The listing builds one solid part. Answer for the finished solid, in the listing's coordinates (mm). A direction names the side the tool comes from. Give positions to 0.01 mm unless a question says otherwise; leave off trailing zeros. Write each loop counter-clockwise with the first axis right and the second up, starting at its lowest first coordinate (ties: lowest second). Pieces come first, ordered by that corner, then holes. Notation, with made-up numbers: (-6, 75.5) - (15, 75.5) arc R24 cw to (15, 112.5) - close; hole circle Ø9 at (61, 80.5). An arc over 180 degrees is marked (long way). Return JSON: item names as keys, results as strings.
from build123d import *

# Parameters (mm, degrees)
SKETCH_1_W           = 20
SKETCH_1_H           = 19
SKETCH_1_R           = 7.5
EXTRUDE_3_DEPTH      = 5
EXTRUDE_4_DEPTH      = 0.0001
EXTRUDE_4_DEPTH_BACK = 5
SKETCH_3_W           = 5
SKETCH_3_H           = 2
SKETCH_4_R           = 1.5
CUT_EXTRUDE_1_DEPTH  = 25.718414189
SKETCH_5_R           = 1.5
CUT_EXTRUDE_2_DEPTH  = 25.718414189
SKETCH_6_W           = 5.334039958
SKETCH_6_H           = 1
CUT_EXTRUDE_3_DEPTH  = 19.445893852


with BuildPart() as part:
    # 草图1 → 凸台-拉伸3 (new body)
    with BuildSketch(Plane(origin=(0, 0, 0), x_dir=(0, 0, -1), z_dir=(1, 0, 0))):
        Rectangle(SKETCH_1_W, SKETCH_1_H)
        Circle(SKETCH_1_R, mode=Mode.SUBTRACT)
    extrude(amount=EXTRUDE_3_DEPTH)

    # 草图3 → 凸台-拉伸4 (add, two sides: drawn at the far end of the back side and taken through both)
    with BuildSketch(Plane.ZY.offset(-EXTRUDE_4_DEPTH_BACK)):
        with Locations((12.5, 8.5)):
            Rectangle(SKETCH_3_W, SKETCH_3_H)
        with Locations((12.5, -8.5)):
            Rectangle(SKETCH_3_W, SKETCH_3_H)
        with Locations((-12.5, 8.5)):
            Rectangle(SKETCH_3_W, SKETCH_3_H)
        with Locations((-12.5, -8.5)):
            Rectangle(SKETCH_3_W, SKETCH_3_H)
    extrude(amount=EXTRUDE_4_DEPTH + EXTRUDE_4_DEPTH_BACK)

    # 草图4 → 切除-拉伸1 (cut, through all)
    with BuildSketch(Plane(origin=(0, 9.5, 0), x_dir=(1, 0, 0), z_dir=(0, 1, 0))):
        with Locations(Location((2.49995, -12.5, 0), (0, 0, 270))):
            Circle(SKETCH_4_R)
    extrude(amount=-CUT_EXTRUDE_1_DEPTH, mode=Mode.SUBTRACT)

    # 草图5 → 切除-拉伸2 (cut, through all)
    with BuildSketch(Plane(origin=(0, 9.5, 0), x_dir=(1, 0, 0), z_dir=(0, 1, 0))):
        with Locations(Location((2.49995, 12.5, 0), (0, 0, 270))):
            Circle(SKETCH_5_R)
    extrude(amount=-CUT_EXTRUDE_2_DEPTH, mode=Mode.SUBTRACT)

    # 草图6 → 切除-拉伸3 (cut, through all)
    with BuildSketch(Plane(origin=(5, 0, 0), x_dir=(0, 0, -1), z_dir=(1, 0, 0))):
        with Locations((-7.5, 0)):
            Rectangle(SKETCH_6_W, SKETCH_6_H)
    extrude(amount=-CUT_EXTRUDE_3_DEPTH, mode=Mode.SUBTRACT)


solid = part.part
Item 1: A cutting plane is placed at B-B on x = 3. Give the number of separate pieces and of enclosed holes in the cut face, then the cut area to 3 significant figures.
Answer below:
{"separate pieces": "5", "enclosed holes": "0", "area": "218 mm²"}
Item 2: A cutting plane is placed at A-A on z = 4.5. Determine the outline of the cut face in (x, y).
Answer below:
{"outline": "(0, -9.5) - (5, -9.5) - (5, -6) - (0, -6) - close; (0, 6) - (5, 6) - (5, 9.5) - (0, 9.5) - close"}
Item 3: Consider L1, parallel to X at y = -8.6, z = 12.5; L2, parallel to Y at x = 3.75, z = 8; L3, parallel to Z at x = 3.4, y = 8.75. Determine where each line is inside the solid, lowest interval first.
Answer below:
{"L1": "x = 0 to 1, 4 to 5", "L2": "y = -9.5 to -0.5, 0.5 to 9.5", "L3": "z = -15 to -13.7, -11.3 to 11.3, 13.7 to 15"}
Item 4: The mould has two halves that part along X. Classify faces 4 (the face through (0, -8, -13)), 5 (the face through (2.57, -8.49, 11)), 6 (the face through (3, 0.5, 9)): +X half, -X half, draft (parallel to the pull), parting line (faces both ways), or undercut.
Answer below:
{"face 4": "-X half", "face 5": "undercut", "face 6": "draft"}
Item 5: For faces 1 (the face through (2, 0, -10)), 2 (the face through (0, -8, 12)), 3 (the face through (4, -7.5, 11)), determine the directions among +Z, -Z, +X, -X, +Y, -Y from which every point of the face is accessible in a straight line to the end or side of a thin tool.
Answer below:
{"face 1": "-Z, +X, -X", "face 2": "+Z, -Z, -X, +Y, -Y", "face 3": "+Z, +X, -X"}
Item 6: A cutting plane is placed at D-D on y = -7. Determine the outline of the cut face in (x, z).
Answer below:
{"outline": "(0, -10) - (5, -10) - (5, -2.69) - (0, -2.69) - close; (0, 2.69) - (5, 2.69) - (5, 10) - (0, 10) - close"}
Item 7: A cutting plane is placed at C-C on z = 12.5. Determine the outline of the cut face in (x, y).
Answer below:
{"outline": "(0, -9.5) - (1, -9.5) - (1, -7.5) - (0, -7.5) - close; (0, 7.5) - (1, 7.5) - (1, 9.5) - (0, 9.5) - close; (4, -9.5) - (5, -9.5) - (5, -7.5) - (4, -7.5) - close; (4, 7.5) - (5, 7.5) - (5, 9.5) - (4, 9.5) - close"}
Item 8: Flat-ended cylindrical pins translate along their axes: P1, Ø1.5, axis at x = 3.5, z = -11.5, coming from the +Y side; P2, Ø1.8, axis at x = 2.5, z = -12.5, coming from the -Y side; P3, Ø1.5, axis at x = 3.5, y = 3, coming from the +Z side; P4, Ø1.5, axis at x = 2, y = 0, coming from the -Z side. Find the tip coordinate at first contact, or state that the pin passes through.
Answer below:
{"P1": "stops at y = 9.5", "P2": "passes through", "P3": "stops at z = 10", "P4": "stops at z = -10"}
